Could you check a few things on this drawing? It's one solid part, dimensions in mm from its lowest x, y, z. Round coordinates to 2 decimals unless told otherwise and drop trailing zeros. Order: outer loops, then holes, each group sorted by start corner. A loop starts at its lowest first (then second) coordinate and runs counter-clockwise, first axis right, second up. Notation, with made-up numbers: (48, 23) - (67, 23) arc R31 ccw to (67, 52) - close; hole circle Ø9 at (54.5, 7.25). An arc over 180 degrees is marked (long way). Use one line per item in the form item = value.
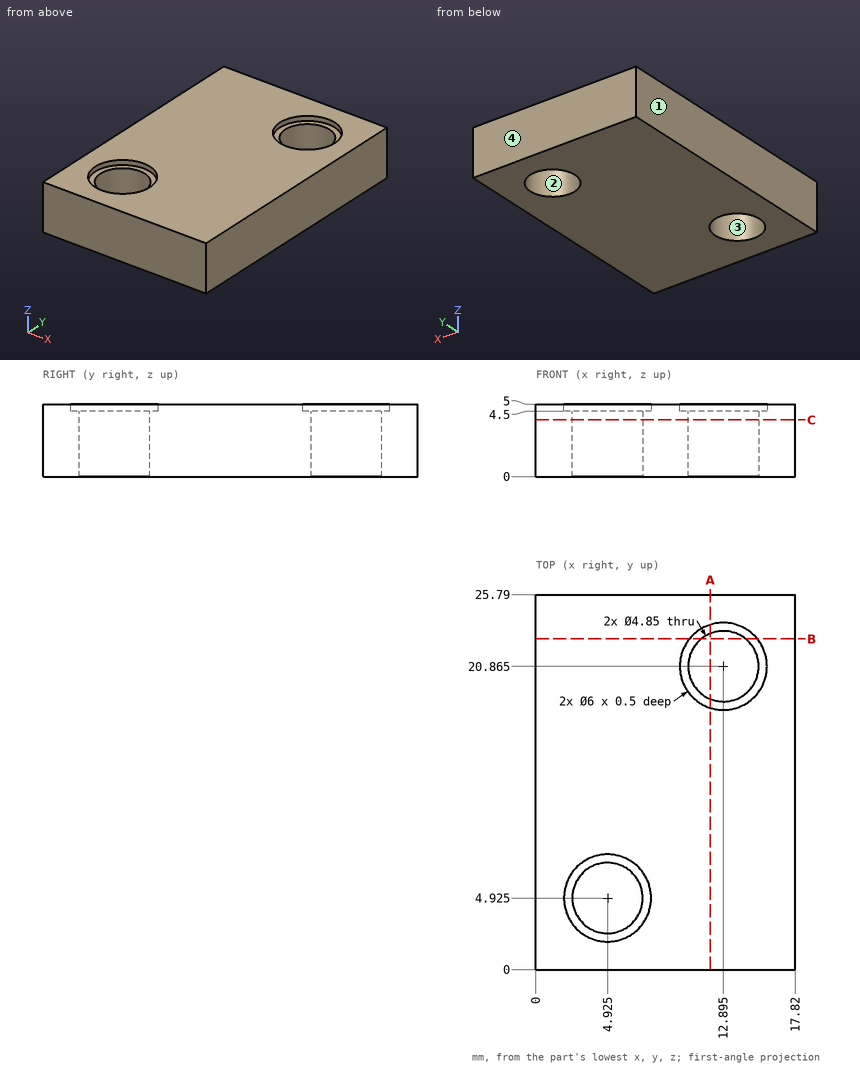
Item 1: Imagine slicing it at B-B on y = 22.75. Please give me the cut outline in (x, z).
Found:
outline = (0, 0) - (11.37, 0) - (11.37, 4.5) - (10.56, 4.5) - (10.56, 5) - (0, 5) - close; (14.42, 0) - (17.82, 0) - (17.82, 5) - (15.23, 5) - (15.23, 4.5) - (14.42, 4.5) - close
Item 2: Imagine slicing it at A-A on x = 12. Please give me the cut outline in (y, z), plus the area to 3 significant figures.
Found:
outline = (0, 0) - (18.61, 0) - (18.61, 4.5) - (18, 4.5) - (18, 5) - (0, 5) - close; (23.12, 0) - (25.79, 0) - (25.79, 5) - (23.73, 5) - (23.73, 4.5) - (23.12, 4.5) - close
area = 106 mm2
Item 3: If we mould it in two halves opening along Y, with no side actions, what happens to the marked faces 1, 2, 3 and 4? For each: released by +Y, released by -Y, zero draft, split by the parting line, or undercut.
Found:
face_1 = zero draft
face_2 = undercut
face_3 = undercut
face_4 = released by +Y
Item 4: I need wall thicknesses on L1, parallel to X at y = 20.75, z = 0.2; L2, parallel to Y at x = 12.75, z = 0.7; L3, parallel to Y at x = 5, z = 2.55. Which ranges of each line are inside material? Lowest first, please.
Found:
L1 = 0 to 10.47, 15.32 to 17.82
L2 = 0 to 18.44, 23.29 to 25.79
L3 = 0 to 2.5, 7.35 to 25.79
Item 5: Imagine slicing it at C-C on z = 3.9. Please give me the cut outline in (x, y) (3 decimals), plus the area to 3 significant figures.
Found:
outline = (0, 0) - (17.82, 0) - (17.82, 25.79) - (0, 25.79) - close; hole circle Ø4.85 at (4.925, 4.925); hole circle Ø4.85 at (12.895, 20.865)
area = 423 mm2
Item 6: Will these pins go through, and if not, where does the flat tip stop? P1, Ø3, axis at x = 5.5, y = 5.5, coming from the +Z side; P2, Ø3, axis at x = 7, y = 21.5, coming from the -Z side.
Found:
P1 = through
P2 = 0
